Design review of the part shown in the three views and the two pictorial views. Dimensions are in mm from the part's minimum x, y and z. Give positions to 0.01 mm unless a question says otherwise; leave off trailing zeros. Loops run counter-clockwise (first coordinate to the right, second up) from the corner with the lowest first, then second, coordinate; pieces in that order, holes last.
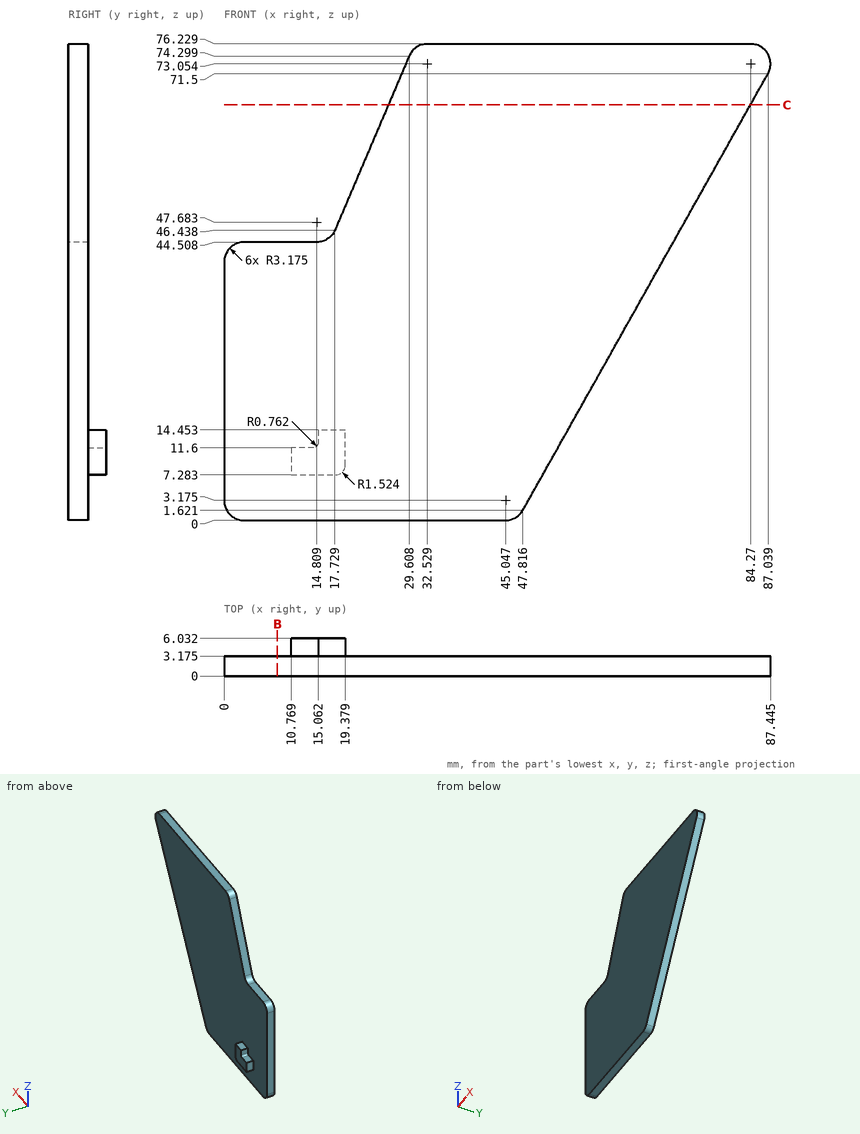
Q1. Take a section at C-C (z = 66.5). Give the boundary of the cut face in (x, y) (1 decimal).
Results:
outline: (26.3, 0) - (84.2, 0) - (84.2, 3.2) - (26.3, 3.2) - close
Q2. Wall thickness on line 1 (Y direction, x = 83, z = 66.5) (1 decimal); line 2 (Z direction, x = 5.5, y = 2); line 3 (Z direction, x = 16, y = 4): over which ranges is each line inside the solid? List them lowest first.
Results:
line 1: y = 0 to 3.2
line 2: z = 0 to 44.51
line 3: z = 7.28 to 14.45
Q3. Insertion check: pin 1 (1.4 mm diameter, centred on y = 4, z = 10.5, fed in from +X); pin 2 (6 mm diameter, centred on x = 37.5, z = 36, fed in from +Y) (1 decimal); pin 3 (1.4 mm diameter, centred on y = 4, z = 8.5, fed in from -X). Each pin has a flat end and moves straight along its axis. Give the tip position at first contact, or say it passes through.
Results:
pin 1: stops at x = 19.38
pin 2: stops at y = 3.2
pin 3: stops at x = 10.77
Q4. Take a section at B-B (x = 8.5). Give the boundary of the cut face in (y, z) (1 decimal), plus the area to 3 significant figures.
Results:
outline: (0, 0) - (3.2, 0) - (3.2, 44.5) - (0, 44.5) - close
area: 141 mm2
